Read the model definition and answer for the solid it produces. Units are mm, in the model's axes. Face numbers are marked on the shaded views. Coordinates: 2 decimals unless noted, no trailing zeros. Order: outer loops, then holes, each group sorted by start corner. A loop starts at its lowest first (then second) coordinate and runs counter-clockwise, first axis right, second up. Notation, with made-up numbers: (37, -37.5) - (49, -37.5) arc R32 cw to (49, -1.5) - close; hole circle Ø7 at (17.25, 56). An arc over 180 degrees is marked (long way). Use one line per item in the form item = value.
```python
from build123d import *

# Parameters (mm, degrees)
SKETCH_R             = 5.75
PAD_DEPTH            = 106
SKETCH001_R          = 1
POCKET_DEPTH         = 20
POCKET_DEPTH_BACK    = -20
PAD001_DEPTH         = 1
SKETCH003_R          = 1
POCKET001_DEPTH      = 20
POCKET001_DEPTH_BACK = -20
SKETCH005_R          = 4
POCKET003_DEPTH      = 5
POCKET003_DEPTH_BACK = 5
SKETCH006_R          = 2
POCKET004_DEPTH      = 50
SKETCH007_W          = 47.595639
SKETCH007_H          = 11
SKETCH007_W_2        = 12.114317
POCKET005_DEPTH      = 20
POCKET005_DEPTH_BACK = -20
SKETCH008_R          = 1.5
POCKET006_DEPTH      = 8.751
SKETCH009_R          = 12.128258
POCKET007_DEPTH      = 16
SKETCH010_R          = 8.873547
SKETCH010_R_2        = 4
POCKET008_DEPTH      = 25


with BuildPart() as part:
    # Sketch → Pad (new body)
    with BuildSketch(Plane.XY):
        Circle(SKETCH_R)
    extrude(amount=PAD_DEPTH)

    # Sketch001 → Pocket (cut, two sides)
    with BuildSketch(Plane.YZ) as pocket_sk:
        with Locations((0, 98.5)):
            Circle(SKETCH001_R)
    extrude(amount=-POCKET_DEPTH, mode=Mode.SUBTRACT)
    extrude(pocket_sk.sketch, amount=-POCKET_DEPTH_BACK, mode=Mode.SUBTRACT)

    # Sketch002 (on Face4 of Pocket) → Pad001 (join)
    with BuildSketch(Plane.XY.offset(106)):
        Polygon((0, 0), (1, 0.57735), (1, 0), align=None)
    extrude(amount=PAD001_DEPTH)

    # Sketch003 (on Face7 of Pad001) → Pocket001 (cut, two sides)
    with BuildSketch(Plane(origin=(0, 0, 0), x_dir=(-0.866026, -0.5, 0), z_dir=(-0.5, 0.866026, 0))) as pocket001_sk:
        with Locations((0, 98.5)):
            Circle(SKETCH003_R)
    extrude(amount=-POCKET001_DEPTH, mode=Mode.SUBTRACT)
    extrude(pocket001_sk.sketch, amount=-POCKET001_DEPTH_BACK, mode=Mode.SUBTRACT)

    # Sketch005 → Pocket003 (cut, two sides)
    with BuildSketch(Plane.XY.offset(106)) as pocket003_sk:
        Circle(SKETCH005_R)
    extrude(amount=POCKET003_DEPTH, mode=Mode.SUBTRACT)
    extrude(pocket003_sk.sketch, amount=-POCKET003_DEPTH_BACK, mode=Mode.SUBTRACT)

    # Sketch006 (on Face3 of Pocket003) → Pocket004 (cut)
    with BuildSketch(Plane.XY.offset(106)):
        Circle(SKETCH006_R)
    extrude(amount=-POCKET004_DEPTH, mode=Mode.SUBTRACT)

    # Sketch007 → Pocket005 (cut, two sides)
    with BuildSketch(Plane.XZ) as pocket005_sk:
        with Locations((-26.797819, 53.75)):
            Rectangle(SKETCH007_W, SKETCH007_H)
        with Locations((9.057158, 53.75)):
            Rectangle(SKETCH007_W_2, SKETCH007_H)
    extrude(amount=-POCKET005_DEPTH, mode=Mode.SUBTRACT)
    extrude(pocket005_sk.sketch, amount=-POCKET005_DEPTH_BACK, mode=Mode.SUBTRACT)

    # Sketch008 (on Face11 of Pocket005) → Pocket006 (cut, through all)
    with BuildSketch(Plane(origin=(-3, 0, 0), x_dir=(0, -1, 0), z_dir=(-1, 0, 0))):
        with Locations((0, 53.75)):
            Circle(SKETCH008_R)
    extrude(amount=-POCKET006_DEPTH, mode=Mode.SUBTRACT)

    # Sketch009 (on Face2 of Pocket006) → Pocket007 (cut)
    with BuildSketch(Plane(origin=(0, 0, 0), x_dir=(1, 0, 0), z_dir=(0, 0, -1))):
        Circle(SKETCH009_R)
    extrude(amount=-POCKET007_DEPTH, mode=Mode.SUBTRACT)

    # Sketch010 (on Face2 of Pocket007) → Pocket008 (cut)
    with BuildSketch(Plane(origin=(0, 0, 16), x_dir=(1, 0, 0), z_dir=(0, 0, -1))):
        Circle(SKETCH010_R)
        Circle(SKETCH010_R_2, mode=Mode.SUBTRACT)
    extrude(amount=-POCKET008_DEPTH, mode=Mode.SUBTRACT)


solid = part.part
```
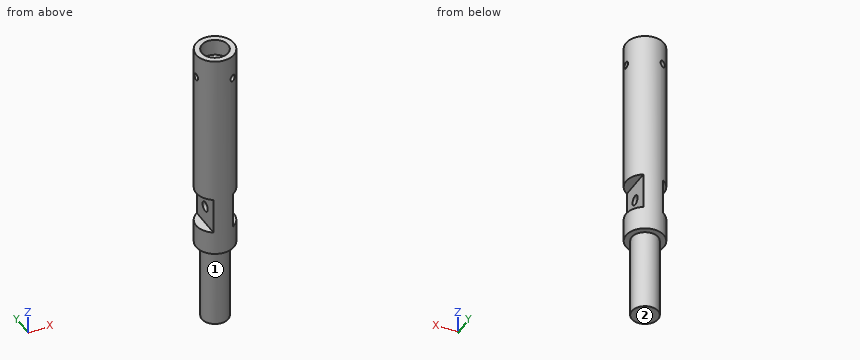
(1) The mould has two halves that part along Y. Classify the marked faces 1 and 2: +Y half, -Y half, draft (parallel to the pull), parting line (faces both ways), or undercut.
Answer list:
face_1 = parting line
face_2 = draft
(2) Straight lines are drawn through the part: L1, parallel to Z at x = 4.8, y = 0; L2, parallel to Z at x = 2.25, y = 0; L3, parallel to Y at x = 0, z = 103.55. For each, find the intervals that lie inside material, in ascending order.
Answer list:
L1 = 41 to 48.25, 59.25 to 97.5, 99.5 to 106
L2 = 16 to 52.25, 55.25 to 97.5, 99.5 to 101
L3 = -5.75 to -4, 4 to 5.75
(3) Section C-C, the plane y = 0 is taken. State how many separate pieces and enclosed holes the cut face has, then the cut area to 3 significant figures.
Answer list:
separate_pieces = 4
enclosed_holes = 0
area = 634 mm2
(4) Section A-A, the plane z = 53.75 is taken. Write down the section's boundary in (x, y), then the cut area to 3 significant figures.
Answer list:
outline = (-3, -4.91) arc R5.75 ccw to (3, -4.91) - (3, -1.5) - (-3, -1.5) - close; (-3, 1.5) - (3, 1.5) - (3, 4.91) arc R5.75 ccw to (-3, 4.91) - close
area = 47.7 mm2
(5) Section B-B, the plane z = 76.5 is taken. Write down the section's boundary in (x, y), then the cut area to 3 significant figures.
Answer list:
outline = circle Ø11.5 at (0, 0); hole circle Ø4 at (0, 0)
area = 91.3 mm2
(6) Section D-D, the plane z = 39.5 is taken. Write down the section's boundary in (x, y).
Answer list:
outline = circle Ø8 at (0, 0)
(7) Given pin 1 Ø5 at (y, z) = (1.5, 52.5) entering from +X; pin 2 Ø2 at (x, z) = (2, 52) entering from +Y; pin 3 Ø6 at (y, z) = (1.5, 27.5) entering from +X, each flat-ended and moving along its own axis, determine where each tip first touches the part or whether it passes through.
Answer list:
pin_1 = 3
pin_2 = 5.66
pin_3 = 4
